from build123d import *

# Parameters (mm, degrees)
SKETCH1_W           = 40
SKETCH1_H           = 40
BOSS_EXTRUDE1_DEPTH = 5
CUT_EXTRUDE1_DEPTH  = 3
SKETCH3_R           = 1.4
CUT_EXTRUDE2_DEPTH  = 3
FILLET1_R           = 5
SKETCH3_3_R         = 2.4
SKETCH3_3_R_2       = 1.4
BOSS_EXTRUDE2_DEPTH = 13.9


with BuildPart() as part:
    # Sketch1 → Boss-Extrude1 (new body)
    with BuildSketch(Plane(origin=(0, 0, 0), x_dir=(1, 0, 0), z_dir=(0, 1, 0))):
        Rectangle(SKETCH1_W, SKETCH1_H)
    extrude(amount=BOSS_EXTRUDE1_DEPTH)

    # Sketch2 → Cut-Extrude1 (cut)
    with BuildSketch(Plane(origin=(0, 5, 0), x_dir=(1, 0, 0), z_dir=(0, 1, 0))):
        Polygon((-6.766838493, 10), (-8.383419246, 12.8), (-11.616580754, 12.8), (-13.233161507, 10), (-11.616580754, 7.2), (-8.383419246, 7.2), align=None)
        Polygon((13.233161507, 10), (11.616580754, 12.8), (8.383419246, 12.8), (6.766838493, 10), (8.383419246, 7.2), (11.616580754, 7.2), align=None)
        Polygon((-6.766838493, -10), (-8.383419246, -7.2), (-11.616580754, -7.2), (-13.233161507, -10), (-11.616580754, -12.8), (-8.383419246, -12.8), align=None)
        Polygon((13.233161507, -10), (11.616580754, -7.2), (8.383419246, -7.2), (6.766838493, -10), (8.383419246, -12.8), (11.616580754, -12.8), align=None)
    extrude(amount=-CUT_EXTRUDE1_DEPTH, mode=Mode.SUBTRACT)

    # Sketch3 → Cut-Extrude2 (cut, through all)
    with BuildSketch(Plane(origin=(0, 2, 0), x_dir=(1, 0, 0), z_dir=(0, 1, 0))):
        with Locations((-10, 10)):
            Circle(SKETCH3_R)
        with Locations((10, -10)):
            Circle(SKETCH3_R)
        with Locations((10, 10)):
            Circle(SKETCH3_R)
        with Locations((-10, -10)):
            Circle(SKETCH3_R)
    extrude(amount=-CUT_EXTRUDE2_DEPTH, mode=Mode.SUBTRACT)

    # Fillet1
    fillet1_edges = [part.edges().sort_by_distance(p)[0] for p in [
        (20, 2.5, 20),
        (-20, 2.5, 20),
        (-20, 2.5, -20),
        (20, 2.5, -20),
    ]]
    fillet(fillet1_edges, radius=FILLET1_R)

    # Sketch3_3 → Boss-Extrude2 (add)
    with BuildSketch(Plane(origin=(0, 2, 0), x_dir=(1, 0, 0), z_dir=(0, 1, 0))):
        with Locations((-10, 10)):
            Circle(SKETCH3_3_R)
        with Locations((-10, 10)):
            Circle(SKETCH3_3_R_2, mode=Mode.SUBTRACT)
        with Locations((-10, -10)):
            Circle(SKETCH3_3_R)
        with Locations((-10, -10)):
            Circle(SKETCH3_3_R_2, mode=Mode.SUBTRACT)
        with Locations((10, -10)):
            Circle(SKETCH3_3_R)
        with Locations((10, -10)):
            Circle(SKETCH3_3_R_2, mode=Mode.SUBTRACT)
        with Locations((10, 10)):
            Circle(SKETCH3_3_R)
        with Locations((10, 10)):
            Circle(SKETCH3_3_R_2, mode=Mode.SUBTRACT)
    extrude(amount=-BOSS_EXTRUDE2_DEPTH)


solid = part.part
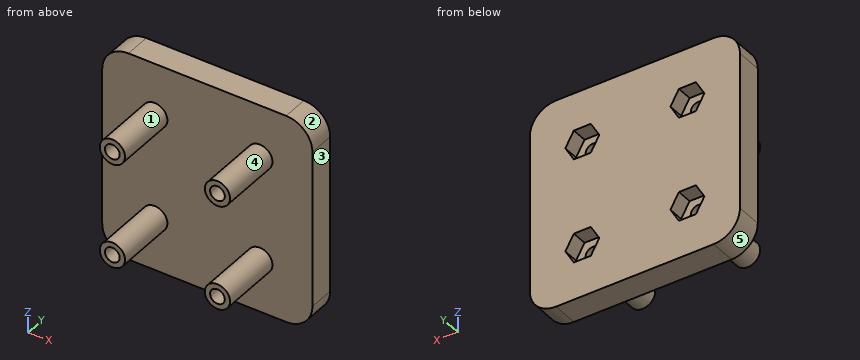
The listing builds one solid part. Answer for the finished solid, in the listing's coordinates (mm). Face numbers are marked on the shaded views. A direction names the side the tool comes from. Coordinates: 2 decimals unless noted, no trailing zeros. Loops run counter-clockwise (first coordinate to the right, second up) from the corner with the lowest first, then second, coordinate; pieces in that order, holes last. Notation, with made-up numbers: M 63,-4 L 80,-4 A35 cw 80,31 Z; hole C 17,-32 d9. An arc over 180 degrees is marked long. Answer in a Markdown table with one row per item.
1) Find section C-C (y = 1). Determine the outline of the cut face in (x, z).
Answers below:
| item | result |
|---|---|
| outline | M -20,-15 A5 ccw -15,-20 L 15,-20 A5 ccw 20,-15 L 20,15 A5 ccw 15,20 L -15,20 A5 ccw -20,15 Z; hole C -10,-10 d2.8; hole C -10,10 d2.8; hole C 10,-10 d2.8; hole C 10,10 d2.8 |
2) Determine the mould class of the marked faces 1, 2 and 3 for opening direction Z: released by +Z, released by -Z, zero draft, split by the parting line, or undercut.
Answers below:
| item | result |
|---|---|
| face 1 | undercut |
| face 2 | released by +Z |
| face 3 | zero draft |
3) Given pin 1 (3 mm diameter, centred on x = -8.5, z = -9.5, fed in from +Y); pin 2 (4 mm diameter, centred on x = -13.5, y = -2.5, fed in from +Z); pin 3 (3 mm diameter, centred on x = 10, z = 10, fed in from +Y), each flat-ended and moving along its own axis, determine where each tip first touches the part or whether it passes through.
Answers below:
| item | result |
|---|---|
| pin 1 | y = 5 |
| pin 2 | z = 11.87 |
| pin 3 | y = 2 |
4) Which of the six approach directions +Z, -Z, +X, -X, +Y, -Y give full straight-line access (tool end or side, diameter ignored) to the marked faces 4 and 5?
Answers below:
| item | result |
|---|---|
| face 4 | -Y |
| face 5 | -Z, -X, +Y, -Y |
5) Find section B-B (x = 10). Determine the outline of the cut face in (y, z).
Answers below:
| item | result |
|---|---|
| outline | M -11.9,-12.4 L 0,-12.4 L 0,-20 L 5,-20 L 5,-12.8 L 2,-12.8 L 2,-11.4 L -11.9,-11.4 Z; M -11.9,-8.6 L 2,-8.6 L 2,-7.2 L 5,-7.2 L 5,7.2 L 2,7.2 L 2,8.6 L -11.9,8.6 L -11.9,7.6 L 0,7.6 L 0,-7.6 L -11.9,-7.6 Z; M -11.9,11.4 L 2,11.4 L 2,12.8 L 5,12.8 L 5,20 L 0,20 L 0,12.4 L -11.9,12.4 Z |
6) Find section D-D (z = 3). Determine the outline of the cut face in (x, y), then the cut area to 3 significant figures.
Answers below:
| item | result |
|---|---|
| outline | M -20,0 L 20,0 L 20,5 L -20,5 Z |
| area | 200 mm^2 |
7) Find the intervals of material crossed by probe 1 along X at (y, z) = (-5.5, -10); probe 2 along Z at (x, y) = (11, -4), in increasing order.
Answers below:
| item | result |
|---|---|
| probe 1 | -12.4 to -11.4, -8.6 to -7.6, 7.6 to 8.6, 11.4 to 12.4 |
| probe 2 | -12.18 to -10.98, -9.02 to -7.82, 7.82 to 9.02, 10.98 to 12.18 |
8) Find section A-A (y = -9.5). Determine the outline of the cut face in (x, z).
Answers below:
| item | result |
|---|---|
| outline | C -10,-10 d4.8; C -10,10 d4.8; C 10,-10 d4.8; C 10,10 d4.8; hole C -10,-10 d2.8; hole C -10,10 d2.8; hole C 10,-10 d2.8; hole C 10,10 d2.8 |
